Geometry: see drawing. Coordinates: mm, zero at the bounding-box minimum. A direction names the side the tool comes from. Give positions to 0.01 mm unless a question says otherwise; leave off trailing zeros. Write each loop counter-clockwise with the first axis right and the second up, starting at its lowest first coordinate (ties: lowest second). Pieces come first, ordered by that corner, then holes. Notation, with made-up numbers: (89.5, 74.25) - (132.5, 74.25) arc R11 cw to (132.5, 94.25) - close; hole circle Ø6 at (3.5, -24). An arc over 180 degrees is marked (long way). Use a Markdown table: item, result. Add a question column.
1. Material intervals for probe 1 along Y at (x, z) = (20, 141); probe 2 along Z at (x, y) = (34.5, 8.5); probe 3 along Z at (x, y) = (21, 22.5), sorted ascending.
2. Section query D-D, the plane y = 28.5. Return loops of the section in (x, z).
3. Pin query (flat end, axial travel): pin 1 (4 mm diameter, centred on y = 32.5, z = 108, fed in from -X); pin 2 (11 mm diameter, centred on x = 20, y = 20, fed in from -Z); pin 3 (10 mm diameter, centred on x = 11.5, z = 56.5, fed in from -Y). Return the tip coordinate at first contact, or that it passes through.
4. Set-up query: the marked faces 1, 2 and 3. Return all of +Z, -Z, +X, -X, +Y, -Y with unobstructed straight access to the full face (end or side cutting, diameter ignored); none if empty.
5. Section query C-C, the plane z = 20. Return loops of the section in (x, y).
6. Section query A-A, the plane x = 20. Return loops of the section in (y, z), plus the area to 3 significant figures.
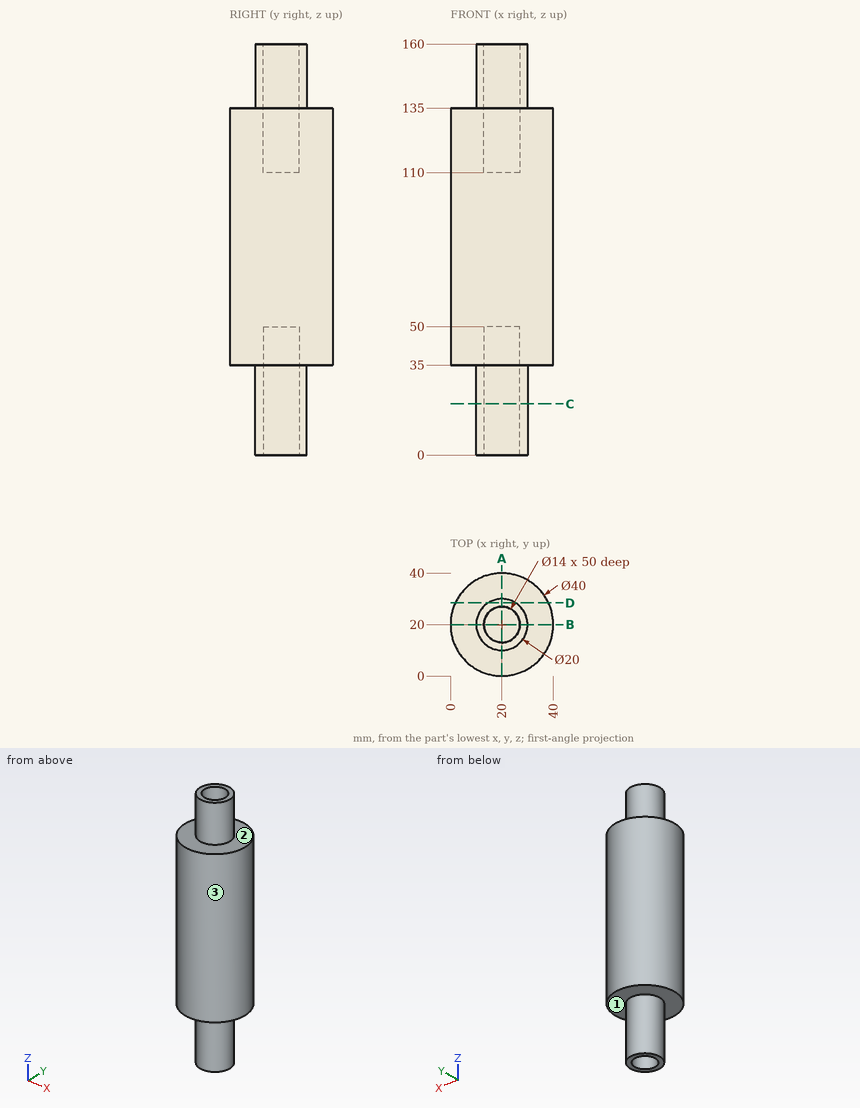
Result sheet:
| question | item | result |
|---|---|---|
| 1 | probe 1 | y = 10 to 13, 27 to 30 |
| 1 | probe 2 | z = 35 to 135 |
| 1 | probe 3 | z = 50 to 110 |
| 2 | outline | (1.9, 35) - (14.73, 35) - (14.73, 0) - (25.27, 0) - (25.27, 35) - (38.1, 35) - (38.1, 135) - (25.27, 135) - (25.27, 160) - (14.73, 160) - (14.73, 135) - (1.9, 135) - close |
| 3 | pin 1 | stops at x = 2.98 |
| 3 | pin 2 | stops at z = 50 |
| 3 | pin 3 | stops at y = 0.31 |
| 4 | face 1 | -Z |
| 4 | face 2 | +Z |
| 4 | face 3 | +Z, -Z |
| 5 | outline | circle Ø20 at (20, 20); hole circle Ø14 at (20, 20) |
| 6 | outline | (0, 35) - (10, 35) - (10, 0) - (13, 0) - (13, 50) - (27, 50) - (27, 0) - (30, 0) - (30, 35) - (40, 35) - (40, 135) - (30, 135) - (30, 160) - (27, 160) - (27, 110) - (13, 110) - (13, 160) - (10, 160) - (10, 135) - (0, 135) - close |
| 6 | area | 3,800 mm² |
